Verification items for the finished model (mm, model axes). Coordinates: 2 decimals unless noted, no trailing zeros. Write each loop counter-clockwise with the first axis right and the second up, starting at its lowest first coordinate (ties: lowest second). Pieces come first, ordered by that corner, then holes. Notation, with made-up numbers: (34.25, 18.5) -> (65.25, 18.5) arc R7 ccw to (65.25, 26.5) -> close; hole circle Ø10 at (-14, 32.25). An arc over 180 degrees is marked (long way). Write each question's results on one line, items separated by ' | '. Start each with the question number.
from build123d import *

# Parameters (mm, degrees)
F0_R     = 3
F1_DEPTH = 3
F2_SIZE  = 1
F3_SIZE  = 2


with BuildPart() as f1:
    # F0 (on Front) → F1 (new body)
    with BuildSketch(Plane.XZ):
        with BuildLine():
            ThreePointArc((0, -5), (-3.535534, 3.535534), (5, 0))
            ThreePointArc((5, 0), (15, -10), (25, 0))
            ThreePointArc((25, 0), (0, 25), (-25, 0))
            ThreePointArc((-25, 0), (-23.826115, -4.701031), (-20.580062, -8.298368))
            Line((-20.580062, -8.298368), (-17.955888, -10.062938))
            ThreePointArc((-17.955888, -10.062938), (-12.696811, -15.52306), (-10.152199, -22.664192))
            Line((-10.152199, -22.664192), (-10.126959, -22.857049))
            Line((-10.126959, -22.857049), (-5.949267, -54.778603))
            ThreePointArc((-5.949267, -54.778603), (-3.957801, -58.509524), (0, -60))
            Line((0, -60), (0, -5))
        make_face()
        with Locations((-15, 0)):
            Circle(F0_R, mode=Mode.SUBTRACT)
        with Locations((15, 0)):
            Circle(F0_R, mode=Mode.SUBTRACT)
        with BuildLine():
            ThreePointArc((-10.128077, -22.856554), (-10.127518, -22.856802), (-10.126959, -22.857049))
            Line((-10.126959, -22.857049), (-10.152199, -22.664192))
            ThreePointArc((-10.152199, -22.664192), (-10.139879, -22.760341), (-10.128077, -22.856554))
        make_face()
    extrude(amount=F1_DEPTH)

    # F2
    f2_edges = [f1.edges().sort_by_distance(p)[0] for p in [
        (-18, -3, 0),
        (12, -3, 0),
    ]]
    chamfer(f2_edges, length=F2_SIZE)

    # F3
    f3_edges = [f1.edges().sort_by_distance(p)[0] for p in [
        (0, -3, -32.5),
    ]]
    chamfer(f3_edges, length=F3_SIZE)


solid = f1.part
1. Sectioned sample at B-B on z = 15. Record the cut outline in (x, y).
2. Material ranges on probe 1 along Z at (x, y) = (0, -1.1); probe 2 along Z at (x, y) = (-13, -0.3); probe 3 along X at (y, z) = (-2.6, -7), recorded low to high. Write a range as from..to.
3. Mould release check, pull along Z, two halves, no side actions. Record for faces 1 (the flat face through (-6, -3, 2)), 2 (the cylindrical face through (12, -1, 0)), 3 (the cylindrical face through (15, -1, -10)): +Z half, -Z half, draft (parallel to the pull), parting line (faces both ways), or undercut.
4. Sectioned sample at A-A on x = 15. Record the cut outline in (y, z).
5. Sectioned sample at D-D on z = 6. Record the cut outline in (x, y), plus the area to 3 significant figures.
6. Sectioned sample at C-C on x = -15. Record the cut outline in (y, z), plus the area to 3 significant figures.
7. Depth check by flat-ended pin: pin 1 Ø1 at (x, y) = (18, -2) entering from +Z; pin 2 Ø5 at (x, z) = (15, 0) entering from -Y; pin 3 Ø1 at (x, y) = (10.5, -2.5) entering from +Z; pin 4 Ø1.1 at (y, z) = (-0.5, -45.5) entering from +X. Enter the tip coordinate at first touch or a pass-through.
Computed values:
1) outline: (-20, -3) -> (20, -3) -> (20, 0) -> (-20, 0) -> close
2) probe 1: z = 5..25 | probe 2: z = -15.05..-2.24, 2.24..21.35 | probe 3: x = -22.14..-1.6, 7.86..22.14
3) face 1: draft | face 2: undercut | face 3: -Z half
4) outline: (-3, -10) -> (0, -10) -> (0, -3) -> (-2, -3) -> (-3, -4) -> close; (-3, 4) -> (-2, 3) -> (0, 3) -> (0, 20) -> (-3, 20) -> close
5) outline: (-24.27, -3) -> (24.27, -3) -> (24.27, 0) -> (-24.27, 0) -> close | area: 146 mm^2
6) outline: (-3, -12.55) -> (0, -12.55) -> (0, -3) -> (-2, -3) -> (-3, -4) -> close; (-3, 4) -> (-2, 3) -> (0, 3) -> (0, 20) -> (-3, 20) -> close | area: 78.7 mm^2
7) pin 1: stops at z = 17.85 | pin 2: passes through | pin 3: stops at z = 22.91 | pin 4: stops at x = 0
